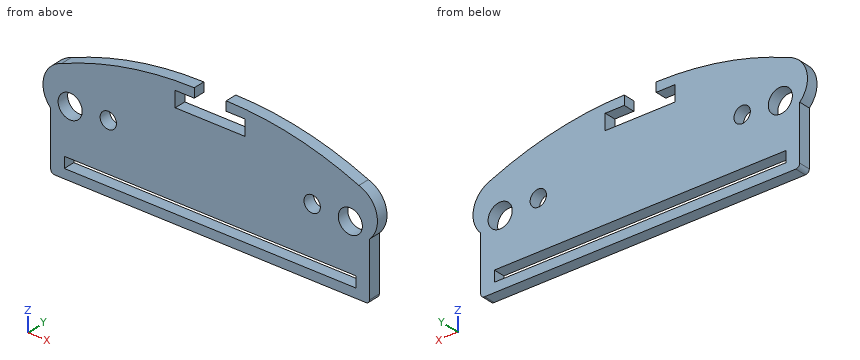
```python
from build123d import *

# Parameters (mm, degrees)
F0_W      = 43
F0_H      = 16.6
F1_DEPTH  = 0.75
F2_W      = 37.5
F2_H      = 1.4
F3_DEPTH  = 75
F5_R      = 1.05
F5_R_2    = 1.55
F6_DEPTH  = 1.501
F7_W      = 4.1
F7_H      = 1.9489285067
F7_H_2    = 0.8016004696
F7_W_2    = 2
F7_H_3    = 15
F8_DEPTH  = 1.501
F10_DEPTH = 1.501
F11_R     = 0.5


# Not quite as in the source:
# - a feature of the source that left no trace in its solid (it failed there, or was rolled back) is left out
# - a pattern or mirror of a feature is missing from the dataset's text; its kind, count and spacing are read off the source's solid


with BuildPart() as f1:
    # F0 (on Front) → F1 (new body, symmetric)
    with BuildSketch(Plane.XZ):
        Rectangle(F0_W, F0_H)
    extrude(amount=F1_DEPTH, both=True)

    # F2 (on Front) → F3 (cut, symmetric)
    with BuildSketch(Plane.XZ):
        with Locations((0, -6.4)):
            Rectangle(F2_W, F2_H)
    extrude(amount=F3_DEPTH, both=True, mode=Mode.SUBTRACT)

    # F5 (on face) → F6 (cut, through all)
    with BuildSketch(Plane.XZ.offset(0.75)):
        with Locations((13.1, 0.5)):
            Circle(F5_R)
        with Locations((18, 0.3)):
            Circle(F5_R_2)
    f6 = extrude(amount=-F6_DEPTH, mode=Mode.SUBTRACT)

    # F6_copies: F6 across plane
    add(f6.mirror(Plane(origin=(0, 0, 0), x_dir=(0, 0, -1), z_dir=(-1, 0, 0))), mode=Mode.SUBTRACT)

    # F7 (on face) → F8 (cut, through all)
    with BuildSketch(Plane.XZ.offset(0.75)):
        Polygon((-2.05, 7.1), (-4.5, 7.1), (-4.5, 5.1), (4.5, 5.1), (4.5, 7.1), (2.05, 7.1), (2.05, 6.2983995304), (-2.05, 6.2983995304), align=None)
        with Locations((0, 8.0744642533)):
            Rectangle(F7_W, F7_H)
        with Locations((0, 6.6991997652)):
            Rectangle(F7_W, F7_H_2)
        with Locations((21.5, -8.3)):
            Rectangle(F7_W_2, F7_H_3)
    f8 = extrude(amount=-F8_DEPTH, mode=Mode.SUBTRACT)

    # F8_copies: F8 across plane
    add(f8.mirror(Plane(origin=(0, 0, 0), x_dir=(0, 0, -1), z_dir=(-1, 0, 0))), mode=Mode.SUBTRACT)

    # F9 (on face) → F10 (cut, through all)
    with BuildSketch(Plane.XZ.offset(0.75)):
        with BuildLine():
            ThreePointArc((2.05, 8.3), (10.75214793, 7.4237307967), (19.104892388, 4.8301066272))
            ThreePointArc((19.104892388, 4.8301066272), (21.392838702, 2.4091433089), (20.5, -0.8))
            Line((20.5, -0.8), (29.8848059028, -7.0995693095))
            Line((29.8848059028, -7.0995693095), (22.5688572973, 15.8109050244))
            Line((22.5688572973, 15.8109050244), (2.05, 8.3))
        make_face()
    f10 = extrude(amount=-F10_DEPTH, mode=Mode.SUBTRACT)

    # F10_copies: F10 across plane
    add(f10.mirror(Plane(origin=(0, 0, 0), x_dir=(0, 0, -1), z_dir=(-1, 0, 0))), mode=Mode.SUBTRACT)

    # F11
    f11_edges = [f1.edges().sort_by_distance(p)[0] for p in [
        (20.5, 0, -8.3),
        (-20.5, 0, -8.3),
    ]]
    fillet(f11_edges, radius=F11_R)


solid = f1.part
```
Check sheet for the modelled part. Datum: model origin and axes. Units: mm. Coordinates: 2 decimals unless noted, no trailing zeros. Order: outer loops, then holes, each group sorted by start corner. A loop starts at its lowest first (then second) coordinate and runs counter-clockwise, first axis right, second up. Notation, with made-up numbers: M -10.75,23 L 23.25,23 A7 cw 23.25,32 Z; hole C 7,71.5 d4. An arc over 180 degrees is marked long. One line per question, with ' | ' between items. Start each with the question number.
Item 1: Sectioned sample at C-C on y = 0.25. Record the cut outline in (x, z).
Item 2: Material ranges on line 1 (Z direction, x = 13.1, y = 0.25); line 2 (Z direction, x = -18, y = -0.1); line 3 (Z direction, x = 10.5, y = 0.25), recorded low to high.
Item 3: Sectioned sample at B-B on x = -18. Record the cut outline in (y, z), and give its area (3 significant figures).
Item 4: Sectioned sample at D-D on x = 7.5. Record the cut outline in (y, z), and give its area (3 significant figures).
Item 5: Sectioned sample at A-A on z = 5.5. Record the cut outline in (x, y).
Item 6: Gauge pin test, flat ends, axial feed: P1, Ø5, axis at x = 18, z = 0.3, coming from the -Y side; P2, Ø1.9, axis at x = -13.1, z = 0.5, coming from the -Y side. Record the tip position at first contact, or that the pin passes through.
Answer below:
1) outline: M -20.5,-7.8 A0.5 ccw -20,-8.3 L 20,-8.3 A0.5 ccw 20.5,-7.8 L 20.5,-0.8 A3.39 ccw 19.1,4.83 A43.65 ccw 2.05,8.3 L 2.05,7.1 L 4.5,7.1 L 4.5,5.1 L -4.5,5.1 L -4.5,7.1 L -2.05,7.1 L -2.05,8.3 A43.65 ccw -19.1,4.83 A3.39 ccw -20.5,-0.8 Z; hole C -18,0.3 d3.1; hole M -18.75,-7.1 L 18.75,-7.1 L 18.75,-5.7 L -18.75,-5.7 Z; hole C -13.1,0.5 d2.1; hole C 13.1,0.5 d2.1; hole C 18,0.3 d3.1
2) line 1: z = -8.3 to -7.1, -5.7 to -0.55, 1.55 to 6.88 | line 2: z = -8.3 to -7.1, -5.7 to -1.25, 1.85 to 5.28 | line 3: z = -8.3 to -7.1, -5.7 to 7.47
3) outline: M -0.75,-8.3 L 0.75,-8.3 L 0.75,-7.1 L -0.75,-7.1 Z; M -0.75,-5.7 L 0.75,-5.7 L 0.75,-1.25 L -0.75,-1.25 Z; M -0.75,1.85 L 0.75,1.85 L 0.75,5.28 L -0.75,5.28 Z | area: 13.6 mm^2
4) outline: M -0.75,-8.3 L 0.75,-8.3 L 0.75,-7.1 L -0.75,-7.1 Z; M -0.75,-5.7 L 0.75,-5.7 L 0.75,7.96 L -0.75,7.96 Z | area: 22.3 mm^2
5) outline: M -17.43,-0.75 L -4.5,-0.75 L -4.5,0.75 L -17.43,0.75 Z; M 4.5,-0.75 L 17.43,-0.75 L 17.43,0.75 L 4.5,0.75 Z
6) P1: stops at y = -0.75 | P2: passes through
